```python
from build123d import *

# Parameters (mm, degrees)
F0_W         = 51.0475635529
F0_H         = 34.7123146057
F1_DEPTH     = 25
F2_R         = 5
F3_T1_DEPTH  = 50
F3_T3_DEPTH  = 76.0475635529
F4_T1_DEPTH  = 41.0475635528
F4_T3_DEPTH  = 24.7123146058
F4_S7_W      = 5
F4_S7_H      = 5
F4_T8_DEPTH  = 5
F4_S13_W     = 5
F4_S13_H     = 5
F4_T14_DEPTH = 5
F4_T18_ANGLE = 90.0000000014
F4_T20_ANGLE = 90.0000000014
F5_T1_DEPTH  = 49.7123146058


# Not quite as in the source:
# - a fillet or chamfer that OpenCascade refuses, or shapes differently, is made with other operations: its cross-section is extruded or revolved along the edge and cut away or added


with BuildPart() as f1:
    # F0 (on Front) → F1 (new body)
    with BuildSketch(Plane.XZ):
        Rectangle(F0_W, F0_H)
    extrude(amount=F1_DEPTH)

    # F2
    f2_edges = [f1.edges().sort_by_distance(p)[0] for p in [
        (0, -25, 17.356157),
        (0, 0, 17.356157),
        (-25.523782, -12.5, 17.356157),
        (25.523782, -12.5, 17.356157),
    ]]
    fillet(f2_edges, radius=F2_R)

    # F3: fillet of radius 5 on 4 edges, made by hand

    # F3_s2 → F3_t1 (cut)
    with BuildSketch(Plane.XZ.offset(-12.5)):
        with BuildLine():
            ThreePointArc((-25.5237817764, -12.3561573029), (-24.0593156824, -15.8916912088), (-20.5237817764, -17.3561573029))
            Line((-20.5237817764, -17.3561573029), (-25.5237817764, -17.3561573029))
            Line((-25.5237817764, -17.3561573029), (-25.5237817764, -12.3561573029))
        make_face()
        with BuildLine():
            ThreePointArc((25.5237817764, -12.3561573029), (24.0593156824, -15.8916912088), (20.5237817764, -17.3561573029))
            Line((20.5237817764, -17.3561573029), (25.5237817764, -17.3561573029))
            Line((25.5237817764, -17.3561573029), (25.5237817764, -12.3561573029))
        make_face()
    extrude(amount=F3_T1_DEPTH, mode=Mode.SUBTRACT)

    # F3_s4 → F3_t3 (cut)
    with BuildSketch(Plane.YZ.offset(-38.0237817764)):
        with BuildLine():
            ThreePointArc((-25, -12.3561573029), (-23.5355339059, -15.8916912088), (-20, -17.3561573029))
            Line((-20, -17.3561573029), (-25, -17.3561573029))
            Line((-25, -17.3561573029), (-25, -12.3561573029))
        make_face()
    extrude(amount=F3_T3_DEPTH, mode=Mode.SUBTRACT)

    # F4: fillet of radius 5 on 3 edges, made by hand

    # F4_s2 → F4_t1 (cut)
    with BuildSketch(Plane.YZ.offset(-20.5237817764)):
        with BuildLine():
            ThreePointArc((0, -12.3561573029), (-1.4644660941, -15.8916912088), (-5, -17.3561573029))
            Line((-5, -17.3561573029), (0, -17.3561573029))
            Line((0, -17.3561573029), (0, -12.3561573029))
        make_face()
    extrude(amount=F4_T1_DEPTH, mode=Mode.SUBTRACT)

    # F4_s4 → F4_t3 (cut)
    with BuildSketch(Plane.XY.offset(-12.3561573029)):
        with BuildLine():
            ThreePointArc((25.5237817764, -5), (24.0593156824, -1.4644660941), (20.5237817764, 0))
            Line((20.5237817764, 0), (25.5237817764, 0))
            Line((25.5237817764, 0), (25.5237817764, -5))
        make_face()
        with BuildLine():
            ThreePointArc((-25.5237817764, -5), (-24.0593156824, -1.4644660941), (-20.5237817764, 0))
            Line((-20.5237817764, 0), (-25.5237817764, 0))
            Line((-25.5237817764, 0), (-25.5237817764, -5))
        make_face()
    extrude(amount=F4_T3_DEPTH, mode=Mode.SUBTRACT)


with BuildPart() as f4_tool6:
    # F4_s7 → F4_t8 (new body)
    with BuildSketch(Plane.YZ.offset(20.5237817764)):
        with Locations((-2.5, 14.8561573029)):
            Rectangle(F4_S7_W, F4_S7_H)
    extrude(amount=F4_T8_DEPTH)

    # F4_s9 → F4_t10 (revolve, cut)
    with BuildSketch(Plane(origin=(20.5237817764, -5, 12.3561573029), x_dir=(0, -0.7071067812, -0.7071067812), z_dir=(0, -0.7071067812, 0.7071067812))):
        with BuildLine():
            ThreePointArc((0, -5), (5, 0), (0, 5))
            Line((0, 5), (0, -5))
        make_face()
    revolve(axis=Axis((20.5237817764, -5, 12.3561573029), (1, 0, 0)), mode=Mode.SUBTRACT)


with BuildPart() as f1_1:
    add(f1.part)

    # F4_t5: cut F4_tool6
    add(f4_tool6.part, mode=Mode.SUBTRACT)


with BuildPart() as f4_tool12:
    # F4_s13 → F4_t14 (new body)
    with BuildSketch(Plane.YZ.offset(-20.5237817764)):
        with Locations((-2.5, 14.8561573029)):
            Rectangle(F4_S13_W, F4_S13_H)
    extrude(amount=-F4_T14_DEPTH)

    # F4_s15 → F4_t16 (revolve, cut)
    with BuildSketch(Plane(origin=(-20.5237817764, -5, 12.3561573029), x_dir=(0, -0.7071067812, -0.7071067812), z_dir=(0, 0.7071067812, -0.7071067812))):
        with BuildLine():
            ThreePointArc((0, -5), (5, 0), (0, 5))
            Line((0, 5), (0, -5))
        make_face()
    revolve(axis=Axis((-20.5237817764, -5, 12.3561573029), (-1, 0, 0)), mode=Mode.SUBTRACT)


with BuildPart() as f1_2:
    add(f1_1.part)

    # F4_t11: cut F4_tool12
    add(f4_tool12.part, mode=Mode.SUBTRACT)

    # F4_s17 → F4_t18 (revolve, cut)
    with BuildSketch(Plane.YZ.offset(-20.5237817765)):
        with BuildLine():
            ThreePointArc((0, -12.3561573029), (-1.4644660941, -15.8916912088), (-5, -17.3561573029))
            Line((-5, -17.3561573029), (0, -17.3561573029))
            Line((0, -17.3561573029), (0, -12.3561573029))
        make_face()
    revolve(axis=Axis((-20.5237817765, 0, -12.356157303), (0, 1, 0)), revolution_arc=F4_T18_ANGLE, mode=Mode.SUBTRACT)

    # F4_s19 → F4_t20 (revolve, cut)
    with BuildSketch(Plane.XY.offset(-12.356157303)):
        with BuildLine():
            ThreePointArc((20.5237817764, 0), (24.0593156823, -1.4644660941), (25.5237817764, -5))
            Line((25.5237817764, -5), (25.5237817764, 0))
            Line((25.5237817764, 0), (20.5237817764, 0))
        make_face()
    revolve(axis=Axis((20.5237817765, 0, -12.356157303), (0, 1, 0)), revolution_arc=F4_T20_ANGLE, mode=Mode.SUBTRACT)

    # F5: fillet of radius 5 on 4 edges, made by hand

    # F5_s2 → F5_t1 (cut)
    with BuildSketch(Plane.XY.offset(-24.8561573029)):
        with BuildLine():
            ThreePointArc((20.5237817764, -25), (24.0593156824, -23.5355339059), (25.5237817764, -20))
            Line((25.5237817764, -20), (25.5237817764, -25))
            Line((25.5237817764, -25), (20.5237817764, -25))
        make_face()
        with BuildLine():
            ThreePointArc((-20.5237817764, -25), (-24.0593156824, -23.5355339059), (-25.5237817764, -20))
            Line((-25.5237817764, -20), (-25.5237817764, -25))
            Line((-25.5237817764, -25), (-20.5237817764, -25))
        make_face()
    extrude(amount=F5_T1_DEPTH, mode=Mode.SUBTRACT)


solid = f1_2.part
```
CAD build for the part. Positions are in the model's coordinates, mm. Coordinates: 2 decimals unless noted, no trailing zeros. Order: outer loops, then holes, each group sorted by start corner. A loop starts at its lowest first (then second) coordinate and runs counter-clockwise, first axis right, second up. Notation, with made-up numbers: (8.25, 67.25) - (24.25, 67.25) arc R24 ccw to (24.25, 96.25) - close; hole circle Ø7 at (57, -14). An arc over 180 degrees is marked (long way). Use a Markdown table: item, result. Add a question column.
(1) Flat gauge pin, fed straight in: pin 1 (10 mm diameter, centred on x = -5.5, y = -21.5, fed in from -Z). Where does the tip first touch, or does it go through?
(2) Saw through at B-B (y = -3.25). Give the cut face in (x, z), then the cut area to 3 significant figures.
(3) Saw through at A-A (x = 14). Give the cut face in (y, z).
(4) Drill centre lines: line 1 along X through (y, z) = (-21.5, -0.5); line 2 along Z through (x, y) = (-0.5, -3); line 3 along Z through (x, y) = (-18.5, -21.25). Where is each one in solid material? Low to high. Write a range as [from, to].
Solved:
| question | item | result |
|---|---|---|
| 1 | pin 1 | stops at z = -17.36 |
| 2 | outline | (-25.21, -12.36) arc R4.68 ccw to (-20.52, -17.04) - (20.52, -17.04) arc R4.68 ccw to (25.21, -12.36) - (25.21, 12.36) arc R4.68 ccw to (20.52, 17.04) - (-20.52, 17.04) arc R4.68 ccw to (-25.21, 12.36) - close |
| 2 | area | 1,700 mm² |
| 3 | outline | (-25, -12.36) arc R5 ccw to (-20, -17.36) - (-5, -17.36) arc R5 ccw to (0, -12.36) - (0, 12.36) arc R5 ccw to (-5, 17.36) - (-20, 17.36) arc R5 ccw to (-25, 12.36) - close |
| 4 | line 1 | x = [-25.29, 25.29] |
| 4 | line 2 | z = [-16.94, 16.94] |
| 4 | line 3 | z = [-17.2, 17.2] |
